For this review, take the finished solid that the model builds, in its own axes (mm). Face numbers are marked on the shaded views. A direction names the side the tool comes from. Coordinates: 2 decimals unless noted, no trailing zeros. Loops run counter-clockwise (first coordinate to the right, second up) from the corner with the lowest first, then second, coordinate; pieces in that order, holes last. Notation, with made-up numbers: (18, 50) - (39, 50) arc R26 cw to (39, 71) - close; hole circle Ø5 at (43.25, -38). An arc over 180 degrees is marked (long way). Use one line per item in the form item = value. Start each with the question number.
1. Draft analysis for pull direction Y (two halves, no side actions). For the marked faces 4, 5 and 6, state which applies: +Y half, -Y half, draft (parallel to the pull), parting line (faces both ways), or undercut.
2. Add section A-A on y = 51.5. Give the boundary of the cut face in (x, z), and give its area (3 significant figures).
3. Add section B-B on z = 51.5. Give the boundary of the cut face in (x, y), and give its area (3 significant figures).
4. To check wall thickness, follow probe 1 along Y at (x, z) = (17, 52.5); probe 2 along X at (y, z) = (36.5, 10); probe 3 along Y at (x, z) = (13.5, 43.5). State the ranges of each line that lie inside material, in increasing order.
5. For pin 1 Ø2 at (x, z) = (-5, 22) entering from +Y; pin 2 Ø1.3 at (x, y) = (29.5, 25.5) entering from +Z; pin 3 Ø6 at (x, y) = (17, -19) entering from +Z, all flat-tipped, find the tip position at first contact; note any pin that passes through.
6. Machinability: for the marked faces 1, 2 and 3, which of the approach directions +Z, -Z, +X, -X, +Y, -Y give a long, thin tool a straight path to every point of the face, cutting with its end or side? Answer none if there is none.
7. Add section C-C on x = -5. Give the boundary of the cut face in (y, z).
8. Add section D-D on y = 15.5. Give the boundary of the cut face in (x, z), and give its area (3 significant figures).
```python
from build123d import *

# Parameters (mm, degrees)
F0_W     = 66.675
F0_H     = 88.9
F1_DEPTH = 57.15
F2_T     = -1.27
F4_DEPTH = 5.08
F5_W     = 66.675
F5_H     = 12.7
F6_DEPTH = 1
F7_W     = 66.675
F7_H     = 12.6965791702
F8_DEPTH = 1
F9_DEPTH = 25.4


with BuildPart() as f1:
    # F0 (on Top) → F1 (new body)
    with BuildSketch(Plane.XY):
        with Locations((-1.1231470853, 10.8568438743)):
            Rectangle(F0_W, F0_H)
    extrude(amount=F1_DEPTH)

    # F2
    f2_openings = [f1.faces().sort_by_distance(p)[0] for p in [
        (-1.123147, 10.856844, 57.15),
    ]]
    offset(amount=F2_T, openings=f2_openings)

    # F3 (on face) → F4 (join)
    with BuildSketch(Plane.XY.offset(1.27)):
        Polygon((30.9443529147, 41.3368438743), (28.4043529147, 41.3368438743), (28.4043529147, -0.1921561257), (28.4043529147, -3.3671561257), (28.4043529147, -9.4631561257), (30.9443529147, -9.4631561257), align=None)
        Polygon((-30.6506470853, 41.3368438743), (-33.1906470853, 41.3368438743), (-33.1906470853, -9.4631561257), (-30.6506470853, -9.4631561257), (-30.6506470853, -3.3671561257), (-30.6506470853, -0.1921561257), align=None)
    extrude(amount=F4_DEPTH)

    # F5 (on face) → F6 (join)
    with BuildSketch(Plane(origin=(0, 55.3068438743, 0), x_dir=(-1, 0, 0), z_dir=(0, 1, 0))):
        with Locations((1.1231470853, 50.8)):
            Rectangle(F5_W, F5_H)
    extrude(amount=F6_DEPTH)

    # F7 (on face) → F8 (join)
    with BuildSketch(Plane.XZ.offset(33.5931561257)):
        with Locations((-1.1231470853, 50.8017104149)):
            Rectangle(F7_W, F7_H)
    extrude(amount=F8_DEPTH)

    # F3 (on face) → F9 (cut)
    with BuildSketch(Plane.XY.offset(1.27)):
        Polygon((-33.1906470853, 54.0368438743), (-33.1906470853, 41.3368438743), (-30.6506470853, 41.3368438743), (28.4043529147, 41.3368438743), (30.9443529147, 41.3368438743), (30.9443529147, 54.0368438743), align=None)
    extrude(amount=-F9_DEPTH, mode=Mode.SUBTRACT)


solid = f1.part
```
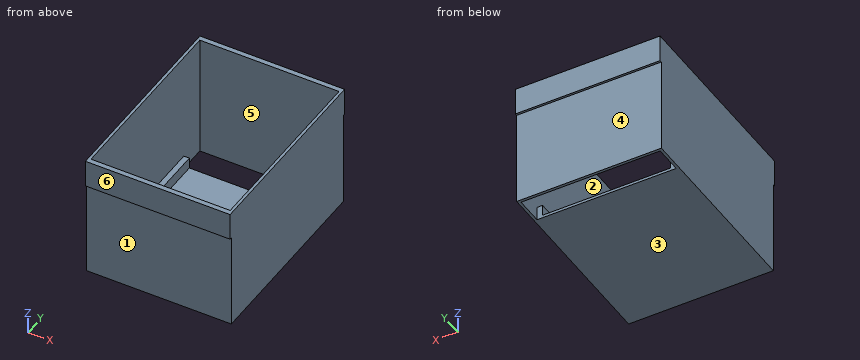
Conclusion:
q1.face_4 = +Y half
q1.face_5 = undercut
q1.face_6 = -Y half
q2.outline = (-34.46, 0) - (-33.19, 0) - (-33.19, 57.15) - (-34.46, 57.15) - close; (30.94, 0) - (32.21, 0) - (32.21, 57.15) - (30.94, 57.15) - close
q2.area = 145 mm^2
q3.outline = (-34.46, -34.59) - (32.21, -34.59) - (32.21, 56.31) - (-34.46, 56.31) - close; hole (-33.19, -32.32) - (30.94, -32.32) - (30.94, 54.04) - (-33.19, 54.04) - close
q3.area = 522 mm^2
q4.probe_1 = -34.59 to -32.32, 54.04 to 56.31
q4.probe_2 = -34.46 to -33.19, 30.94 to 32.21
q4.probe_3 = -33.59 to -32.32, 54.04 to 55.31
q5.pin_1 = 55.31
q5.pin_2 = 6.35
q5.pin_3 = 1.27
q6.face_1 = -Z, +X, -X, -Y
q6.face_2 = +Z
q6.face_3 = -Z, +X, -X, +Y, -Y
q7.outline = (-34.59, 44.45) - (-33.59, 44.45) - (-33.59, 0) - (41.34, 0) - (41.34, 1.27) - (-32.32, 1.27) - (-32.32, 57.15) - (-34.59, 57.15) - close; (54.04, 0) - (55.31, 0) - (55.31, 44.45) - (56.31, 44.45) - (56.31, 57.15) - (54.04, 57.15) - close
q8.outline = (-34.46, 0) - (32.21, 0) - (32.21, 57.15) - (30.94, 57.15) - (30.94, 6.35) - (28.4, 6.35) - (28.4, 1.27) - (-30.65, 1.27) - (-30.65, 6.35) - (-33.19, 6.35) - (-33.19, 57.15) - (-34.46, 57.15) - close
q8.area = 252 mm^2
